```python
from build123d import *

# Parameters (mm, degrees)
SKETCH2_W           = 101.6
SKETCH2_H           = 3.175
BOSS_EXTRUDE1_DEPTH = 199.3
SKETCH3_W           = 101.6
SKETCH3_H           = 199.3
SKETCH3_W_2         = 94.6
SKETCH3_H_2         = 192.95
BOSS_EXTRUDE2_DEPTH = 25.4
SKETCH5_R           = 41.3385
SKETCH5_R_2         = 38.1635
BOSS_EXTRUDE4_DEPTH = 3.175
SKETCH7_R           = 3
SKETCH7_R_2         = 1.375
BOSS_EXTRUDE5_DEPTH = 3.175
SKETCH8_W           = 15.6845
SKETCH8_H           = 15.4686
SKETCH8_W_2         = 15.113
SKETCH8_H_2         = 17.6911
CUT_EXTRUDE1_DEPTH  = 3.175
SKETCH9_R           = 1.375
CUT_EXTRUDE2_DEPTH  = 3.175
SKETCH10_W          = 101.6
SKETCH10_H          = 101.6
CUT_EXTRUDE3_DEPTH  = 7.874


with BuildPart() as part:
    # Sketch2 → Boss-Extrude1 (new body)
    with BuildSketch(Plane.XY):
        with Locations((50.8, 1.5875)):
            Rectangle(SKETCH2_W, SKETCH2_H)
    extrude(amount=BOSS_EXTRUDE1_DEPTH)

    # Sketch3 → Boss-Extrude2 (add)
    with BuildSketch(Plane(origin=(0, 3.175, 0), x_dir=(1, 0, 0), z_dir=(0, 1, 0))):
        with Locations((50.8, -99.65)):
            Rectangle(SKETCH3_W, SKETCH3_H)
        with Locations((50.8, -99.65)):
            Rectangle(SKETCH3_W_2, SKETCH3_H_2, mode=Mode.SUBTRACT)
    extrude(amount=BOSS_EXTRUDE2_DEPTH)

    # Sketch5 → Boss-Extrude4 (add)
    with BuildSketch(Plane(origin=(0, 3.175, 0), x_dir=(1, 0, 0), z_dir=(0, 1, 0))):
        with Locations((50.8, -50.475)):
            Circle(SKETCH5_R)
        with Locations((50.8, -50.475)):
            Circle(SKETCH5_R_2, mode=Mode.SUBTRACT)
    extrude(amount=BOSS_EXTRUDE4_DEPTH)

    # Sketch7 → Boss-Extrude5 (add)
    with BuildSketch(Plane(origin=(0, 3.175, 0), x_dir=(1, 0, 0), z_dir=(0, 1, 0))):
        with Locations((7.127, -172.752)):
            Circle(SKETCH7_R)
        with Locations((7.127, -172.752)):
            Circle(SKETCH7_R_2, mode=Mode.SUBTRACT)
        with Locations((7.127, -114.752)):
            Circle(SKETCH7_R)
        with Locations((7.127, -114.752)):
            Circle(SKETCH7_R_2, mode=Mode.SUBTRACT)
        with Locations((56.127, -172.752)):
            Circle(SKETCH7_R)
        with Locations((56.127, -172.752)):
            Circle(SKETCH7_R_2, mode=Mode.SUBTRACT)
        with Locations((56.127, -114.752)):
            Circle(SKETCH7_R)
        with Locations((56.127, -114.752)):
            Circle(SKETCH7_R_2, mode=Mode.SUBTRACT)
    extrude(amount=BOSS_EXTRUDE5_DEPTH)

    # Sketch8 → Cut-Extrude1 (cut)
    with BuildSketch(Plane.XY.offset(199.3)):
        with Locations((13.425, 14.0843)):
            Rectangle(SKETCH8_W, SKETCH8_H)
        with Locations((32.175, 15.19555)):
            Rectangle(SKETCH8_W_2, SKETCH8_H_2)
        with Locations((50.175, 15.19555)):
            Rectangle(SKETCH8_W_2, SKETCH8_H_2)
    extrude(amount=-CUT_EXTRUDE1_DEPTH, mode=Mode.SUBTRACT)

    # Sketch9 → Cut-Extrude2 (cut)
    with BuildSketch(Plane(origin=(0, 3.175, 0), x_dir=(1, 0, 0), z_dir=(0, 1, 0))):
        with Locations((7.127, -114.752)):
            Circle(SKETCH9_R)
        with Locations((56.127, -114.752)):
            Circle(SKETCH9_R)
        with Locations((56.127, -172.752)):
            Circle(SKETCH9_R)
        with Locations((7.127, -172.752)):
            Circle(SKETCH9_R)
    extrude(amount=-CUT_EXTRUDE2_DEPTH, mode=Mode.SUBTRACT)

    # Sketch10 → Cut-Extrude3 (cut)
    with BuildSketch(Plane(origin=(0, 28.575, 0), x_dir=(1, 0, 0), z_dir=(0, 1, 0))):
        with Locations((50.8, -50.8)):
            Rectangle(SKETCH10_W, SKETCH10_H)
    extrude(amount=-CUT_EXTRUDE3_DEPTH, mode=Mode.SUBTRACT)


solid = part.part
```
Check sheet for the modelled part. Datum: model origin and axes. Units: mm. A direction names the side the tool comes from. Give positions to 0.01 mm unless a question says otherwise; leave off trailing zeros. Loops run counter-clockwise (first coordinate to the right, second up) from the corner with the lowest first, then second, coordinate; pieces in that order, holes last. Notation, with made-up numbers: M 25,31.5 L 51,31.5 A20 ccw 51,63.5 Z; hole C 59.25,9 d2. An arc over 180 degrees is marked long. Answer as CSV lines item,"result".
Item 1: Set-up check for faces 1 (the face through (50, 10, 0)), 2 (the face through (2, 25, 101.6)), 3 (the face through (56, 6.35, 171)): record each of +Z, -Z, +X, -X, +Y, -Y from which the full face is reachable in a straight line by a thin tool's end or side.
Reply:
face 1,"-Z, +X, -X, +Y, -Y"
face 2,"-Z, +X, -X, +Y"
face 3,"+Y"
Item 2: Sectioned sample at D-D, the plane z = 97. Enter the section's corners in (x, y) (3 decimals), then the cut area to 3 significant figures.
Reply:
outline,"M 0,0 L 101.6,0 L 101.6,20.701 L 98.1,20.701 L 98.1,3.175 L 3.5,3.175 L 3.5,20.701 L 0,20.701 Z"
area,"445 mm^2"
Item 3: Scan lines: L1, parallel to X at y = 22.25, z = 124.5; L2, parallel to Z at x = 81, y = 19.5 (3 decimals); L3, parallel to X at y = 5, z = 30.5. Record each from-to range of solid material in increasing order.
Reply:
L1,"0 to 3.5, 98.1 to 101.6"
L2,"0 to 3.175, 196.125 to 199.3"
L3,"0 to 3.5, 14.61 to 18.28, 83.32 to 86.99, 98.1 to 101.6"
Item 4: Sectioned sample at A-A, the plane y = 14.75. Enter the section's corners in (x, z) (1 decimal).
Reply:
outline,"M 0,0 L 101.6,0 L 101.6,199.3 L 57.7,199.3 L 57.7,196.1 L 98.1,196.1 L 98.1,3.2 L 3.5,3.2 L 3.5,196.1 L 5.6,196.1 L 5.6,199.3 L 0,199.3 Z; M 21.3,196.1 L 24.6,196.1 L 24.6,199.3 L 21.3,199.3 Z; M 39.7,196.1 L 42.6,196.1 L 42.6,199.3 L 39.7,199.3 Z"
Item 5: Draft check along Z on faces 4 (the face through (7, 6.35, 171)), 5 (the face through (61, 14, 199.3)), 6 (the face through (100, 25, 101.6)). Enter one of: pulls with the +Z half, pulls with the -Z half, needs draft (parallel to the pull), parting line crosses it, or undercut.
Reply:
face 4,"undercut"
face 5,"pulls with the +Z half"
face 6,"pulls with the -Z half"
Item 6: Sectioned sample at C-C, the plane z = 158.5. Enter the section's corners in (x, y) (3 decimals).
Reply:
outline,"M 0,0 L 101.6,0 L 101.6,28.575 L 98.1,28.575 L 98.1,3.175 L 3.5,3.175 L 3.5,28.575 L 0,28.575 Z"
Item 7: Depth check by flat-ended pin: pin 1 Ø3 at (x, z) = (57.5, 96.5) entering from -Y; pin 2 Ø3 at (x, z) = (55, 172) entering from +Y; pin 3 Ø1.6 at (x, z) = (7.127, 114.752) entering from +Y; pin 4 Ø2 at (x, z) = (32.5, 109) entering from +Y (3 decimals). Enter the tip coordinate at first touch or a pass-through.
Reply:
pin 1,"y = 0"
pin 2,"y = 6.35"
pin 3,"through"
pin 4,"y = 3.175"
